Verification items for the finished model (mm, model axes). Round coordinates to 2 decimals unless told otherwise and drop trailing zeros. Write each loop counter-clockwise with the first axis right and the second up, starting at its lowest first coordinate (ties: lowest second). Pieces come first, ordered by that corner, then holes. Notation, with made-up numbers: (62, -10) - (108, -10) arc R7 cw to (108, 0) - close; hole circle Ø9 at (-25.75, 49.5). An arc over 180 degrees is marked (long way). Answer as a JSON object with one key per item and string values.
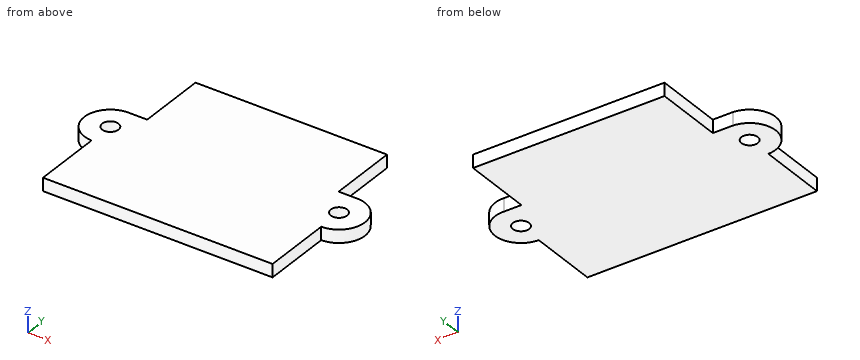
```python
from build123d import *

# Parameters (mm, degrees)
SKETCH1_R           = 0.635000006
BOSS_EXTRUDE1_DEPTH = 1.016


with BuildPart() as part:
    # Sketch1 → Boss-Extrude1 (new body)
    with BuildSketch(Plane.XY):
        with BuildLine():
            Line((-7.4676, 7.430550118), (7.4676, 7.430550118))
            Line((7.4676, 7.430550118), (7.4676, 2.045750118))
            Line((7.4676, 2.045750118), (8.808625011, 2.045750118))
            ThreePointArc((8.808625011, 2.045750118), (10.946108081, 0.089005249), (8.9535, -2.015085385))
            Line((8.9535, -2.015085385), (8.9535, -7.430550118))
            Line((8.9535, -7.430550118), (-8.9535, -7.430550118))
            Line((-8.9535, -7.430550118), (-8.9535, -2.015085385))
            ThreePointArc((-8.9535, -2.015085385), (-10.947109486, -0.017801943), (-9.022174989, 2.045750118))
            Line((-9.022174989, 2.045750118), (-7.4676, 2.045750118))
            Line((-7.4676, 2.045750118), (-7.4676, 7.430550118))
        make_face()
        with Locations((-8.9154, 0.016557396)):
            Circle(SKETCH1_R, mode=Mode.SUBTRACT)
        with Locations((8.9154, 0.016557396)):
            Circle(SKETCH1_R, mode=Mode.SUBTRACT)
    extrude(amount=BOSS_EXTRUDE1_DEPTH)


solid = part.part
```
Q1. Section check D-D, the plane y = 5.5. Record the cut outline in (x, z).
Geometry check:
{"outline": "(-7.47, 0) - (7.47, 0) - (7.47, 1.02) - (-7.47, 1.02) - close"}
Q2. Section check C-C, the plane y = -4. Record the cut outline in (x, z).
Geometry check:
{"outline": "(-8.95, 0) - (8.95, 0) - (8.95, 1.02) - (-8.95, 1.02) - close"}
Q3. Section check B-B, the plane z = 0.3. Record the cut outline in (x, y) (1 decimal), then the cut area to 3 significant figures.
Geometry check:
{"outline": "(-9, -7.4) - (9, -7.4) - (9, -2) arc R2 ccw (long way) to (8.8, 2) - (7.5, 2) - (7.5, 7.4) - (-7.5, 7.4) - (-7.5, 2) - (-9, 2) arc R2 ccw to (-9, -2) - close; hole circle Ø1.3 at (-8.9, 0); hole circle Ø1.3 at (8.9, 0)", "area": "260 mm2"}
Q4. Section check A-A, the plane x = -8.5. Record the cut outline in (y, z).
Geometry check:
{"outline": "(-7.43, 0) - (-0.46, 0) - (-0.46, 1.02) - (-7.43, 1.02) - close; (0.5, 0) - (2.05, 0) - (2.05, 1.02) - (0.5, 1.02) - close"}
Q5. Material ranges on line 1 along X through (y, z) = (4.5, 0.2); line 2 along X through (y, z) = (0.25, 0.5); line 3 along Y through (x, z) = (-9.25, 0.3), recorded low to high. Write a range as [from, to].
Geometry check:
{"line 1": "x = [-7.47, 7.47]", "line 2": "x = [-10.93, -9.51], [-8.32, 8.32], [9.51, 10.93]", "line 3": "y = [-1.99, -0.52], [0.56, 2.02]"}
Q6. Gauge pin test, flat ends, axial feed: P1, Ø2, axis at x = 8.92, y = 0.02, coming from the -Z side; P2, Ø1.1, axis at x = -8.92, y = 0.02, coming from the -Z side. Record the tip position at first contact, or that the pin passes through.
Geometry check:
{"P1": "stops at z = 0", "P2": "passes through"}
